from build123d import *

# Parameters (mm, degrees)
BOSS_EXTRUDE1_DEPTH = 5.9
SKETCH2_W           = 8
SKETCH2_H           = 55
BOSS_EXTRUDE2_DEPTH = 8
SKETCH3_W           = 5.9
SKETCH3_H           = 10
SKETCH3_W_2         = 9
SKETCH3_H_2         = 15
CUT_EXTRUDE1_DEPTH  = 9
BOSS_EXTRUDE3_DEPTH = 5.9
BOSS_EXTRUDE4_DEPTH = 8
SKETCH6_W           = 27.583097586
SKETCH6_H           = 68.456340366
CUT_EXTRUDE2_DEPTH  = 9
BOSS_EXTRUDE5_DEPTH = 5.9
CUT_EXTRUDE3_REACH  = 7.9
SKETCH8_R           = 2.05


with BuildPart() as part:
    # Sketch1 → Boss-Extrude1 (new body)
    with BuildSketch(Plane.XY):
        with BuildLine():
            ThreePointArc((97.061822228, 90.695765473), (82.799132124, 99.447826237), (76.396720763, 83.987165662))
            Line((76.396720763, 83.987165662), (-17.603279237, 83.987165662))
            Line((-17.603279237, 83.987165662), (-17.603279237, 138.987165662))
            Line((-17.603279237, 138.987165662), (94.396720763, 138.987165662))
            Line((94.396720763, 138.987165662), (94.396720763, 110.289306386))
            ThreePointArc((94.396720763, 110.289306386), (103.949970876, 103.334562845), (108.745956392, 92.534953205))
            Line((108.745956392, 92.534953205), (97.061822228, 90.695765473))
        make_face()
    extrude(amount=BOSS_EXTRUDE1_DEPTH)

    # Sketch2 → Boss-Extrude2 (add)
    with BuildSketch(Plane.XY.offset(5.9)):
        with Locations((-21.603279237, 111.487165662)):
            Rectangle(SKETCH2_W, SKETCH2_H)
    extrude(amount=-BOSS_EXTRUDE2_DEPTH)

    # Sketch3 → Cut-Extrude1 (cut, through all)
    with BuildSketch(Plane.XY.offset(5.9)):
        with Locations((91.446720763, 118.987165662)):
            Rectangle(SKETCH3_W, SKETCH3_H)
        with Locations((-21.103279237, 91.487165662)):
            Rectangle(SKETCH3_W_2, SKETCH3_H_2)
    extrude(amount=-CUT_EXTRUDE1_DEPTH, mode=Mode.SUBTRACT)

    # Sketch4 → Boss-Extrude3 (add)
    with BuildSketch(Plane.XY.offset(5.9)):
        Polygon((4.396720763, 138.987165662), (4.396720763, 144.887165662), (-0.603279237, 144.887165662), (-0.603279237, 148.887165662), (19.396720763, 148.887165662), (19.396720763, 144.887165662), (14.396720763, 144.887165662), (14.396720763, 138.987165662), align=None)
        Polygon((49.396720763, 144.887165662), (49.396720763, 148.887165662), (69.396720763, 148.887165662), (69.396720763, 144.887165662), (64.396720763, 144.887165662), (64.396720763, 138.987165662), (54.396720763, 138.987165662), (54.396720763, 144.887165662), align=None)
    extrude(amount=-BOSS_EXTRUDE3_DEPTH)

    # Sketch5 → Boss-Extrude4 (add, through all)
    with BuildSketch(Plane.XY.offset(5.9)):
        Polygon((-25.603279237, 123.987165662), (-33.603279237, 123.987165662), (-33.603279237, 128.987165662), (-37.603279237, 128.987165662), (-37.603279237, 103.987165662), (-33.603279237, 103.987165662), (-33.603279237, 108.987165662), (-25.603279237, 108.987165662), align=None)
    extrude(amount=-BOSS_EXTRUDE4_DEPTH)

    # Sketch6 → Cut-Extrude2 (cut, through all)
    with BuildSketch(Plane.XY.offset(5.9)):
        with Locations((-30.39482803, 118.215335845)):
            Rectangle(SKETCH6_W, SKETCH6_H)
    extrude(amount=-CUT_EXTRUDE2_DEPTH, mode=Mode.SUBTRACT)

    # Sketch7 → Boss-Extrude5 (add)
    with BuildSketch(Plane.XY.offset(5.9)):
        Polygon((-16.603279237, 113.987165662), (-22.503279237, 113.987165662), (-22.503279237, 118.987165662), (-26.503279237, 118.987165662), (-26.503279237, 93.987165662), (-22.503279237, 93.987165662), (-22.503279237, 98.987165662), (-16.603279237, 98.987165662), align=None)
    extrude(amount=-BOSS_EXTRUDE5_DEPTH)

    # Sketch8 → Cut-Extrude3 (cut, up to next)
    with BuildSketch(Plane.XY.offset(5.9), mode=Mode.PRIVATE) as cut_extrude3_sk1:
        with Locations((-16.603279237, 98.987165662)):
            Circle(SKETCH8_R)
    cut_extrude3_tool1 = extrude(cut_extrude3_sk1.sketch, amount=-CUT_EXTRUDE3_REACH, mode=Mode.PRIVATE) & part.part
    add(cut_extrude3_tool1.solids().sort_by_distance((-16.603279, 98.987166, 5.9))[0], mode=Mode.SUBTRACT)
    # Sketch8 → Cut-Extrude3 (cut, up to next)
    with BuildSketch(Plane.XY.offset(5.9), mode=Mode.PRIVATE) as cut_extrude3_sk2:
        with Locations((-22.503279237, 98.987165662)):
            Circle(SKETCH8_R)
    cut_extrude3_tool2 = extrude(cut_extrude3_sk2.sketch, amount=-CUT_EXTRUDE3_REACH, mode=Mode.PRIVATE) & part.part
    add(cut_extrude3_tool2.solids().sort_by_distance((-22.503279, 98.987166, 5.9))[0], mode=Mode.SUBTRACT)
    # Sketch8 → Cut-Extrude3 (cut, up to next)
    with BuildSketch(Plane.XY.offset(5.9), mode=Mode.PRIVATE) as cut_extrude3_sk3:
        with Locations((-22.503279237, 113.987165662)):
            Circle(SKETCH8_R)
    cut_extrude3_tool3 = extrude(cut_extrude3_sk3.sketch, amount=-CUT_EXTRUDE3_REACH, mode=Mode.PRIVATE) & part.part
    add(cut_extrude3_tool3.solids().sort_by_distance((-22.503279, 113.987166, 5.9))[0], mode=Mode.SUBTRACT)
    # Sketch8 → Cut-Extrude3 (cut, up to next)
    with BuildSketch(Plane.XY.offset(5.9), mode=Mode.PRIVATE) as cut_extrude3_sk4:
        with Locations((-16.603279237, 113.987165662)):
            Circle(SKETCH8_R)
    cut_extrude3_tool4 = extrude(cut_extrude3_sk4.sketch, amount=-CUT_EXTRUDE3_REACH, mode=Mode.PRIVATE) & part.part
    add(cut_extrude3_tool4.solids().sort_by_distance((-16.603279, 113.987166, 5.9))[0], mode=Mode.SUBTRACT)
    # Sketch8 → Cut-Extrude3 (cut, up to next)
    with BuildSketch(Plane.XY.offset(5.9), mode=Mode.PRIVATE) as cut_extrude3_sk5:
        with Locations((4.396720763, 138.987165662)):
            Circle(SKETCH8_R)
    cut_extrude3_tool5 = extrude(cut_extrude3_sk5.sketch, amount=-CUT_EXTRUDE3_REACH, mode=Mode.PRIVATE) & part.part
    add(cut_extrude3_tool5.solids().sort_by_distance((4.396721, 138.987166, 5.9))[0], mode=Mode.SUBTRACT)
    # Sketch8 → Cut-Extrude3 (cut, up to next)
    with BuildSketch(Plane.XY.offset(5.9), mode=Mode.PRIVATE) as cut_extrude3_sk6:
        with Locations((14.396720763, 138.987165662)):
            Circle(SKETCH8_R)
    cut_extrude3_tool6 = extrude(cut_extrude3_sk6.sketch, amount=-CUT_EXTRUDE3_REACH, mode=Mode.PRIVATE) & part.part
    add(cut_extrude3_tool6.solids().sort_by_distance((14.396721, 138.987166, 5.9))[0], mode=Mode.SUBTRACT)
    # Sketch8 → Cut-Extrude3 (cut, up to next)
    with BuildSketch(Plane.XY.offset(5.9), mode=Mode.PRIVATE) as cut_extrude3_sk7:
        with Locations((14.396720763, 144.887165662)):
            Circle(SKETCH8_R)
    cut_extrude3_tool7 = extrude(cut_extrude3_sk7.sketch, amount=-CUT_EXTRUDE3_REACH, mode=Mode.PRIVATE) & part.part
    add(cut_extrude3_tool7.solids().sort_by_distance((14.396721, 144.887166, 5.9))[0], mode=Mode.SUBTRACT)
    # Sketch8 → Cut-Extrude3 (cut, up to next)
    with BuildSketch(Plane.XY.offset(5.9), mode=Mode.PRIVATE) as cut_extrude3_sk8:
        with Locations((4.396720763, 144.887165662)):
            Circle(SKETCH8_R)
    cut_extrude3_tool8 = extrude(cut_extrude3_sk8.sketch, amount=-CUT_EXTRUDE3_REACH, mode=Mode.PRIVATE) & part.part
    add(cut_extrude3_tool8.solids().sort_by_distance((4.396721, 144.887166, 5.9))[0], mode=Mode.SUBTRACT)
    # Sketch8 → Cut-Extrude3 (cut, up to next)
    with BuildSketch(Plane.XY.offset(5.9), mode=Mode.PRIVATE) as cut_extrude3_sk9:
        with Locations((54.396720763, 144.887165662)):
            Circle(SKETCH8_R)
    cut_extrude3_tool9 = extrude(cut_extrude3_sk9.sketch, amount=-CUT_EXTRUDE3_REACH, mode=Mode.PRIVATE) & part.part
    add(cut_extrude3_tool9.solids().sort_by_distance((54.396721, 144.887166, 5.9))[0], mode=Mode.SUBTRACT)
    # Sketch8 → Cut-Extrude3 (cut, up to next)
    with BuildSketch(Plane.XY.offset(5.9), mode=Mode.PRIVATE) as cut_extrude3_sk10:
        with Locations((54.396720763, 138.987165662)):
            Circle(SKETCH8_R)
    cut_extrude3_tool10 = extrude(cut_extrude3_sk10.sketch, amount=-CUT_EXTRUDE3_REACH, mode=Mode.PRIVATE) & part.part
    add(cut_extrude3_tool10.solids().sort_by_distance((54.396721, 138.987166, 5.9))[0], mode=Mode.SUBTRACT)
    # Sketch8 → Cut-Extrude3 (cut, up to next)
    with BuildSketch(Plane.XY.offset(5.9), mode=Mode.PRIVATE) as cut_extrude3_sk11:
        with Locations((64.396720763, 138.987165662)):
            Circle(SKETCH8_R)
    cut_extrude3_tool11 = extrude(cut_extrude3_sk11.sketch, amount=-CUT_EXTRUDE3_REACH, mode=Mode.PRIVATE) & part.part
    add(cut_extrude3_tool11.solids().sort_by_distance((64.396721, 138.987166, 5.9))[0], mode=Mode.SUBTRACT)
    # Sketch8 → Cut-Extrude3 (cut, up to next)
    with BuildSketch(Plane.XY.offset(5.9), mode=Mode.PRIVATE) as cut_extrude3_sk12:
        with Locations((64.396720763, 144.887165662)):
            Circle(SKETCH8_R)
    cut_extrude3_tool12 = extrude(cut_extrude3_sk12.sketch, amount=-CUT_EXTRUDE3_REACH, mode=Mode.PRIVATE) & part.part
    add(cut_extrude3_tool12.solids().sort_by_distance((64.396721, 144.887166, 5.9))[0], mode=Mode.SUBTRACT)
    # Sketch8 → Cut-Extrude3 (cut, up to next)
    with BuildSketch(Plane.XY.offset(5.9), mode=Mode.PRIVATE) as cut_extrude3_sk13:
        with Locations((88.496720763, 123.987165662)):
            Circle(SKETCH8_R)
    cut_extrude3_tool13 = extrude(cut_extrude3_sk13.sketch, amount=-CUT_EXTRUDE3_REACH, mode=Mode.PRIVATE) & part.part
    add(cut_extrude3_tool13.solids().sort_by_distance((88.496721, 123.987166, 5.9))[0], mode=Mode.SUBTRACT)
    # Sketch8 → Cut-Extrude3 (cut, up to next)
    with BuildSketch(Plane.XY.offset(5.9), mode=Mode.PRIVATE) as cut_extrude3_sk14:
        with Locations((88.496720763, 113.987165662)):
            Circle(SKETCH8_R)
    cut_extrude3_tool14 = extrude(cut_extrude3_sk14.sketch, amount=-CUT_EXTRUDE3_REACH, mode=Mode.PRIVATE) & part.part
    add(cut_extrude3_tool14.solids().sort_by_distance((88.496721, 113.987166, 5.9))[0], mode=Mode.SUBTRACT)


solid = part.part
Part model, mm, in its own coordinate system. A direction names the side the tool comes from. Round coordinates to 2 decimals unless told otherwise and drop trailing zeros. Loops run counter-clockwise (first coordinate to the right, second up) from the corner with the lowest first, then second, coordinate; pieces in that order, holes last. Notation, with made-up numbers: (-33, -34) - (-23, -34) arc R27 ccw to (-23, -11) - close; hole circle Ø10 at (33, 6). An arc over 180 degrees is marked (long way). Answer as a JSON object with one key per item and string values.
Item 1: Pull direction Y, two halves, no side cores. Call faces 6 (the face through (103.844, 103.464, 2.909)), 7 (the face through (-0.603, 147, 3)), 8 (the face through (-15.11, 100.39, 2.99)): pulls with the +Y half, pulls with the -Y half, needs draft (parallel to the pull), parting line crosses it, or undercut.
Output:
{"face 6": "pulls with the +Y half", "face 7": "needs draft", "face 8": "undercut"}
Item 2: Band-saw the part on B-B on x = 26. List the corners of the cut face in (y, z), plus the area to 4 significant figures.
Output:
{"outline": "(83.99, 0) - (138.99, 0) - (138.99, 5.9) - (83.99, 5.9) - close", "area": "324.5 mm2"}
Item 3: Band-saw the part on A-A on y = 120.5. List the corners of the cut face in (x, z), plus the area to 3 significant figures.
Output:
{"outline": "(-16.6, 0) - (88.5, 0) - (88.5, 5.9) - (-16.6, 5.9) - close", "area": "620 mm2"}
Item 4: Tool access for faces 1 (the face through (-22.503, 95, 3)), 2 (the face through (1, 144.887, 3)), 3 (the face through (-24, 118.987, 3)), 4 (the face through (69.397, 147, 3)), 5 (the face through (19.397, 147, 3)): list every direction of +Z, -Z, +X, -X, +Y, -Y with a clear straight run to the whole face (end or side of a thin tool).
Output:
{"face 1": "+Z, -Z, -Y", "face 2": "+Z, -Z, -X", "face 3": "+Z, -Z, -X, +Y", "face 4": "+Z, -Z, +X, +Y", "face 5": "+Z, -Z, +Y"}
Item 5: Pin check, flat tips, straight feed: pin 1 (3 mm diameter, centred on y = 111.5, z = 4, fed in from +X); pin 2 (2.5 mm diameter, centred on x = -16.6, y = 98.99, fed in from +Z); pin 3 (3 mm diameter, centred on y = 122, z = 4, fed in from -X). Stop position of each tip, or through.
Output:
{"pin 1": "x = 95.11", "pin 2": "through", "pin 3": "x = -16.6"}
Item 6: Wall check: L1, parallel to Y at x = 14.5, z = 2.4; L2, parallel to Y at x = 13.5, z = 0.4; L3, parallel to X at y = 111, z = 2.75. Give the ranges that are in metal, low to high.
Output:
{"L1": "83.99 to 136.94, 146.93 to 148.89", "L2": "83.99 to 137.14, 140.83 to 143.04, 146.73 to 148.89", "L3": "-26.5 to 94.4"}
